from build123d import *

# Parameters (mm, degrees)
F0_W     = 110.9441034496
F0_H     = 56.2861021608
F1_DEPTH = 55.88
F3_DEPTH = 33.02
F4_W     = 71.8694478273
F4_H     = 43.125666678
F5_DEPTH = 10.16
F6_DEPTH = 2.54
F7_DEPTH = 10.16
F8_DEPTH = 2.54


with BuildPart() as f1:
    # F0 (on Top) → F1 (new body)
    with BuildSketch(Plane.XY):
        with Locations((3.2562222332, -4.4191563502)):
            Rectangle(F0_W, F0_H)
    extrude(amount=F1_DEPTH)

    # F2 (on face) → F3 (cut)
    with BuildSketch(Plane.XZ.offset(32.5622074306)):
        Polygon((36.8650741875, 46.9826161861), (-33.3762653172, 46.9826161861), (-5.2332119085, 0), (16.1648113281, 0), align=None)
    extrude(amount=-F3_DEPTH, mode=Mode.SUBTRACT)

    # F4 (on face) → F5 (cut)
    with BuildSketch(Plane.XY.offset(55.88)):
        with Locations((1.1629350483, -10.9993740916)):
            Rectangle(F4_W, F4_H)
    extrude(amount=-F5_DEPTH, mode=Mode.SUBTRACT)

    # F6 (add): a face of the model
    f6_faces = [f1.faces().sort_by_distance(p)[0] for p in [
        (-34.7717888653, -10.9993740916, 50.8),
    ]]
    extrude(f6_faces, amount=F6_DEPTH)

    # F7 (add): a face of the model
    f7_faces = [f1.faces().sort_by_distance(p)[0] for p in [
        (2.4329350483, 10.5634592474, 50.8),
    ]]
    extrude(f7_faces, amount=F7_DEPTH)

    # F8 (add): a face of the model
    f8_faces = [f1.faces().sort_by_distance(p)[0] for p in [
        (37.097658962, -16.0793740916, 50.8),
    ]]
    extrude(f8_faces, amount=F8_DEPTH)


solid = f1.part
The listing builds one solid part. Answer for the finished solid, in the listing's coordinates (mm). A direction names the side the tool comes from. Round coordinates to 2 decimals unless told otherwise and drop trailing zeros. Write each loop counter-clockwise with the first axis right and the second up, starting at its lowest first coordinate (ties: lowest second). Pieces come first, ordered by that corner, then holes. Notation, with made-up numbers: (42.5, -26.5) - (66.5, -26.5) arc R28 ccw to (66.5, -5.5) - close; hole circle Ø3 at (45, 3.5). An arc over 180 degrees is marked (long way). Use one line per item in the form item = value. Start each with the question number.
Item 1: Determine the mould class of faces 3 (the flat face through (2, 23.724, 28)), 4 (the flat face through (1, 0.403, 51)), 5 (the flat face through (-52.216, -5, 28)) for opening direction X: +X half, -X half, draft (parallel to the pull), parting line (faces both ways), or undercut.
Item 2: A cutting plane is placed at A-A (y = -22.5). Write down the section's boundary in (x, z).
Item 3: A cutting plane is placed at B-B (x = 29). Write down the section's boundary in (y, z).
Item 4: A tool of negligible diameter and unlimited length cuts with its end or side. For faces 1 (the flat face through (-32.232, -16, 51)), 2 (the flat face through (42, -32.562, 22)), from which of +Z, -Z, +X, -X, +Y, -Y can it reach the whole face along a straight path? Write none if from no direction.
Item 5: A cutting plane is placed at D-D (x = 9). Write down the section's boundary in (y, z).
Item 6: Find the intervals of material crossed by line 1 (X direction, y = -4.5, z = 46.5); line 2 (Y direction, x = -27, z = 51); line 3 (X direction, y = -26, z = 24), in increasing order. Write a range as [from, to].
Item 7: A cutting plane is placed at C-C (z = 40.5). Write down the section's boundary in (x, y).
Item 8: A flat-ended cylindrical pin translates along its axis: pin 1 Ø5 at (x, z) = (18, 48.5) entering from -Y. Find the tip coordinate at first contact, or state that the pin passes through.
The answers:
q1.face_3 = draft
q1.face_4 = undercut
q1.face_5 = -X half
q2.outline = (-52.22, 0) - (-5.23, 0) - (-32.62, 45.72) - (-32.23, 45.72) - (-32.23, 55.88) - (-52.22, 55.88) - close; (16.16, 0) - (58.73, 0) - (58.73, 55.88) - (34.56, 55.88) - (34.56, 45.72) - (36.31, 45.72) - close
q3.outline = (-32.56, 0) - (23.72, 0) - (23.72, 55.88) - (0.4, 55.88) - (0.4, 45.72) - (0.46, 45.72) - (0.46, 29.13) - (-32.56, 29.13) - close
q4.face_1 = +Z, -Y
q4.face_2 = +Z, -Z, +X, -X, -Y
q5.outline = (0.4, 45.72) - (0.46, 45.72) - (0.46, 0) - (23.72, 0) - (23.72, 55.88) - (0.4, 55.88) - close
q6.line_1 = [-52.22, -32.23], [34.56, 58.73]
q6.line_2 = [0.4, 23.72]
q6.line_3 = [-52.22, -19.61], [26.74, 58.73]
q7.outline = (-52.22, -32.56) - (-29.49, -32.56) - (-29.49, 0.46) - (34.01, 0.46) - (34.01, -32.56) - (58.73, -32.56) - (58.73, 23.72) - (-52.22, 23.72) - close
q8.pin_1 = 0.4
